from build123d import *

# Parameters (mm, degrees)
SKETCH1_W                = 42
SKETCH1_H                = 63
SKETCH1_R                = 11.5
BOSS_EXTRUDE1_DEPTH      = 3.2
M3_CLEARANCE_HOLE1_D     = 3.2
M3_CLEARANCE_SLOT1_DEPTH = 3.2
FILLET1_R                = 1


# Read off the part's stored shape, not the designer's step: M3 Clearance Slot1
with BuildPart() as part:
    # Sketch1 → Boss-Extrude1 (new body)
    with BuildSketch(Plane(origin=(0, 0, 0), x_dir=(1, 0, 0), z_dir=(0, 1, 0))):
        Rectangle(SKETCH1_W, SKETCH1_H)
        with Locations(Location((0, 0, 0), (0, 0, 270))):
            Circle(SKETCH1_R, mode=Mode.SUBTRACT)
    extrude(amount=BOSS_EXTRUDE1_DEPTH)

    # M3 Clearance Hole1 (through all)
    with Locations(Plane(origin=(0, 3.2, 0), x_dir=(1, 0, 0), z_dir=(0, 1, 0))):
        with Locations((-15.5, 15.5), (15.5, 15.5), (15.5, -15.5), (-15.5, -15.5)):
            Hole(M3_CLEARANCE_HOLE1_D / 2)

    # M3 Clearance Slot1 outline → M3 Clearance Slot1 (cut)
    with BuildSketch(Plane(origin=(0, 0, 0), x_dir=(1, 0, 0), z_dir=(0, 1, 0))):
        with BuildLine():
            Line((1.6, -27.75), (1.6, -24.75))
            ThreePointArc((1.6, -24.75), (0, -23.15), (-1.6, -24.75))
            Line((-1.6, -24.75), (-1.6, -27.75))
            ThreePointArc((-1.6, -27.75), (0, -29.35), (1.6, -27.75))
        make_face()
        with BuildLine():
            ThreePointArc((1.6, 27.75), (0, 29.35), (-1.6, 27.75))
            Line((-1.6, 27.75), (-1.6, 24.75))
            ThreePointArc((-1.6, 24.75), (0, 23.15), (1.6, 24.75))
            Line((1.6, 24.75), (1.6, 27.75))
        make_face()
    extrude(amount=M3_CLEARANCE_SLOT1_DEPTH, mode=Mode.SUBTRACT)

    # Fillet1
    fillet1_edges = [part.edges().sort_by_distance(p)[0] for p in [
        (-21, 1.6, -31.5),
        (21, 1.6, -31.5),
        (21, 1.6, 31.5),
        (-21, 1.6, 31.5),
    ]]
    fillet(fillet1_edges, radius=FILLET1_R)


solid = part.part
Input: part model. Units: mm. Frame: model coordinates. A direction names the side the tool comes from. Round coordinates to 2 decimals unless told otherwise and drop trailing zeros. Order: outer loops, then holes, each group sorted by start corner. A loop starts at its lowest first (then second) coordinate and runs counter-clockwise, first axis right, second up. Notation, with made-up numbers: (11, -6.5) - (23, -6.5) arc R9 ccw to (23, -1.5) - close; hole circle Ø11 at (17, 0). An arc over 180 degrees is marked (long way). Answer as a JSON object with one key per item and string values. Group by question number.
(1) Cut plane D-D (z = 15.5). Return loops of the section in (x, y).
(2) Cut plane A-A (x = -15.5). Return loops of the section in (y, z).
(3) Reachability of faces 5 (the face through (0.04, 1.58, -29.35)), 6 (the face through (-10, 3.2, -7)) from +Z, -Z, +X, -X, +Y, -Y: full face, straight path, thin tool, end or side. Return the list, or none.
(4) Material intervals for probe 1 along X at (y, z) = (2.3, -15.5); probe 2 along Z at (x, y) = (-15.5, 2.5); probe 3 along X at (y, z) = (0.7, -16.5), sorted ascending. Write a range as from..to.
(5) Cut plane C-C (x = -7). Return loops of the section in (y, z).
(6) Draft query along Z for faces 1 (the face through (0, 2, -31.5)), 2 (the face through (0, 2, 31.5)), 3 (the face through (9.7, 1.58, 6.18)), 4 (the face through (21, 2, 0)). Return one class per face: released by +Z, released by -Z, zero draft, split by the parting line, or undercut.
(7) Cut plane B-B (z = -26). Return loops of the section in (x, y), then the cut area to 3 significant figures.
Here are the results:
{
 "1": {"outline": "(-21, 0) - (-17.1, 0) - (-17.1, 3.2) - (-21, 3.2) - close; (-13.9, 0) - (13.9, 0) - (13.9, 3.2) - (-13.9, 3.2) - close; (17.1, 0) - (21, 0) - (21, 3.2) - (17.1, 3.2) - close"},
 "2": {"outline": "(0, -31.5) - (3.2, -31.5) - (3.2, -17.1) - (0, -17.1) - close; (0, -13.9) - (3.2, -13.9) - (3.2, 13.9) - (0, 13.9) - close; (0, 17.1) - (3.2, 17.1) - (3.2, 31.5) - (0, 31.5) - close"},
 "3": {"face 5": "+Y, -Y", "face 6": "+Z, -Z, +X, -X, +Y"},
 "4": {"probe 1": "x = -21..-17.1, -13.9..13.9, 17.1..21", "probe 2": "z = -31.5..-17.1, -13.9..13.9, 17.1..31.5", "probe 3": "x = -21..-16.75, -14.25..14.25, 16.75..21"},
 "5": {"outline": "(0, -31.5) - (3.2, -31.5) - (3.2, -9.12) - (0, -9.12) - close; (0, 9.12) - (3.2, 9.12) - (3.2, 31.5) - (0, 31.5) - close"},
 "6": {"face 1": "released by -Z", "face 2": "released by +Z", "face 3": "undercut", "face 4": "zero draft"},
 "7": {"outline": "(-21, 0) - (-1.6, 0) - (-1.6, 3.2) - (-21, 3.2) - close; (1.6, 0) - (21, 0) - (21, 3.2) - (1.6, 3.2) - close", "area": "124 mm^2"}
}
